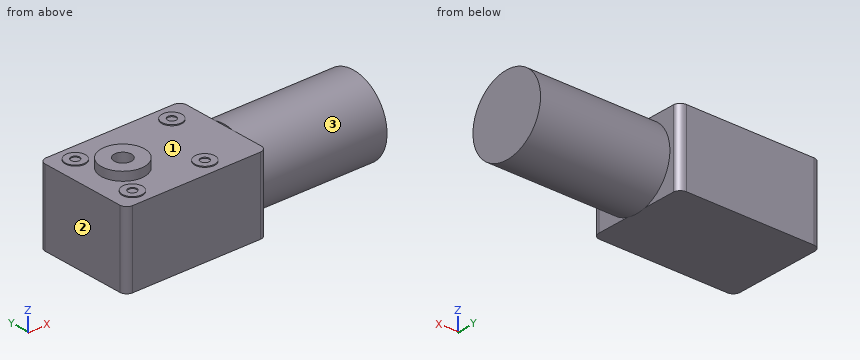
```python
from build123d import *

# Parameters (mm, degrees)
EXTRUDE_1_DEPTH     = 43.5
SKETCH_3_R          = 5.8
SKETCH_3_R_2        = 2.5
EXTRUDE_2_DEPTH     = 0.557471264
SKETCH_3_3_R        = 12.42
SKETCH_3_3_R_2      = 5
EXTRUDE_3_DEPTH     = 5
SKETCH_4_R          = 22.5
EXTRUDE_4_DEPTH     = 75
CUT_EXTRUDE_START   = -10
SKETCH_3_4_R        = 5
CUT_EXTRUDE_1_DEPTH = 10


with BuildPart() as part:
    # Sketch 2 → Extrude 1 (new body)
    with BuildSketch(Plane.XY):
        with BuildLine():
            Line((-37, 28.82), (37, 28.82))
            ThreePointArc((37, 28.82), (39.828427125, 27.648427125), (41, 24.82))
            Line((41, 24.82), (41, -24.82))
            ThreePointArc((41, -24.82), (39.828427125, -27.648427125), (37, -28.82))
            Line((37, -28.82), (-37, -28.82))
            ThreePointArc((-37, -28.82), (-39.828427125, -27.648427125), (-41, -24.82))
            Line((-41, -24.82), (-41, 24.82))
            ThreePointArc((-41, 24.82), (-39.828427125, 27.648427125), (-37, 28.82))
        make_face()
    extrude(amount=EXTRUDE_1_DEPTH)

    # Sketch 3 → Extrude 2 (add)
    # profile 1 of 4: a face of its own
    with BuildSketch(Plane.XY.offset(43.5)):
        with Locations(Location((-28.6, 19, 0), (0, 0, 180))):
            Circle(SKETCH_3_R)
        with Locations((-28.6, 19)):
            Circle(SKETCH_3_R_2, mode=Mode.SUBTRACT)
    # profile 2 of 4: a face of its own
    with BuildSketch(Plane.XY.offset(43.5)):
        with Locations(Location((-28.6, -19, 0), (0, 0, 180))):
            Circle(SKETCH_3_R)
        with Locations((-28.6, -19)):
            Circle(SKETCH_3_R_2, mode=Mode.SUBTRACT)
    # profile 3 of 4: a face of its own
    with BuildSketch(Plane.XY.offset(43.5)):
        with Locations(Location((13.4, -19, 0), (0, 0, 180))):
            Circle(SKETCH_3_R)
        with Locations((13.4, -19)):
            Circle(SKETCH_3_R_2, mode=Mode.SUBTRACT)
    # profile 4 of 4: a face of its own
    with BuildSketch(Plane.XY.offset(43.5)):
        with Locations(Location((27.4, 19, 0), (0, 0, 180))):
            Circle(SKETCH_3_R)
        with Locations((27.4, 19)):
            Circle(SKETCH_3_R_2, mode=Mode.SUBTRACT)
    extrude(amount=EXTRUDE_2_DEPTH)

    # Sketch 3_3 → Extrude 3 (add)
    with BuildSketch(Plane.XY.offset(43.5)):
        with Locations(Location((-17.6, 0, 0), (0, 0, 180))):
            Circle(SKETCH_3_3_R)
        with Locations((-17.6, 0)):
            Circle(SKETCH_3_3_R_2, mode=Mode.SUBTRACT)
    extrude(amount=EXTRUDE_3_DEPTH)

    # Sketch 4 → Extrude 4 (add)
    with BuildSketch(Plane(origin=(41, 0, 0), x_dir=(0, 0, -1), z_dir=(1, 0, 0))):
        with Locations(Location((-21.75, 0, 0), (0, 0, 194.835111582))):
            Circle(SKETCH_4_R)
    extrude(amount=EXTRUDE_4_DEPTH)

    # Sketch 3_4 → Cut-Extrude 1 (cut)
    with BuildSketch(Plane.XY.offset(43.5).offset(CUT_EXTRUDE_START)):
        with Locations((-17.6, 0)):
            Circle(SKETCH_3_4_R)
    extrude(amount=CUT_EXTRUDE_1_DEPTH, mode=Mode.SUBTRACT)


solid = part.part
```
Could you check a few things on this model? Use its own coordinates, in mm. Face numbers are marked on the shaded views. A direction names the side the tool comes from. Give positions to 0.01 mm unless a question says otherwise; leave off trailing zeros. Order: outer loops, then holes, each group sorted by start corner. A loop starts at its lowest first (then second) coordinate and runs counter-clockwise, first axis right, second up.
Q1. If I drill on line 1 along Y through (x, z) = (-28.6, 43.85); line 2 along Y through (x, z) = (-17.6, 37); line 3 along X through (y, z) = (-21, 30.5), over which ranges is the centre line in solid material (lowest first)?
Q2. I'm going to push flat-ended pins straight in: P1, Ø6, axis at x = -27, y = -19.5, coming from the +Z side; P2, Ø4, axis at x = 27.4, y = 19, coming from the -Z side; P3, Ø6, axis at x = -17.6, y = 0, coming from the +Z side. Where does each tip first touch, or does it pass through?
Q3. Suppose I cut it at C-C, the plane z = 28.5. Write out the boundary of the cut face in (x, y), and give its area (3 significant figures).
Q4. Suppose I cut it at A-A, the plane x = 27.4. Write out the boundary of the cut face in (y, z).
Q5. Suppose I cut it at D-D, the plane x = -28.6. Write out the boundary of the cut face in (y, z).
Q6. Suppose I cut it at B-B, the plane y = -19. Write out the boundary of the cut face in (x, z), and give its area (3 significant figures).
Q7. For the marked faces 1, 2 and 3, which set-ups out of +Z, -Z, +X, -X, +Y, -Y let a thin tool reach every point of the face, with its end or its side?
Solution:
1. line 1: y = -24.8 to -21.5, -16.5 to -13.2, -5.77 to 5.77, 13.2 to 16.5, 21.5 to 24.8
1. line 2: y = -28.82 to -5, 5 to 28.82
1. line 3: x = -41 to 41
2. P1: stops at z = 44.06
2. P2: stops at z = 0
2. P3: stops at z = 33.5
3. outline: (-41, -24.82) arc R4 ccw to (-37, -28.82) - (37, -28.82) arc R4 ccw to (41, -24.82) - (41, -21.46) - (116, -21.46) - (116, 21.46) - (41, 21.46) - (41, 24.82) arc R4 ccw to (37, 28.82) - (-37, 28.82) arc R4 ccw to (-41, 24.82) - close
3. area: 7,930 mm2
4. outline: (-28.82, 0) - (28.82, 0) - (28.82, 43.5) - (24.8, 43.5) - (24.8, 44.06) - (21.5, 44.06) - (21.5, 43.5) - (16.5, 43.5) - (16.5, 44.06) - (13.2, 44.06) - (13.2, 43.5) - (-28.82, 43.5) - close
5. outline: (-28.82, 0) - (28.82, 0) - (28.82, 43.5) - (24.8, 43.5) - (24.8, 44.06) - (21.5, 44.06) - (21.5, 43.5) - (16.5, 43.5) - (16.5, 44.06) - (13.2, 44.06) - (13.2, 43.5) - (5.77, 43.5) - (5.77, 48.5) - (-5.77, 48.5) - (-5.77, 43.5) - (-13.2, 43.5) - (-13.2, 44.06) - (-16.5, 44.06) - (-16.5, 43.5) - (-21.5, 43.5) - (-21.5, 44.06) - (-24.8, 44.06) - (-24.8, 43.5) - (-28.82, 43.5) - close
6. outline: (-41, 0) - (41, 0) - (41, 9.7) - (116, 9.7) - (116, 33.8) - (41, 33.8) - (41, 43.5) - (19.2, 43.5) - (19.2, 44.06) - (15.9, 44.06) - (15.9, 43.5) - (10.9, 43.5) - (10.9, 44.06) - (7.6, 44.06) - (7.6, 43.5) - (-22.8, 43.5) - (-22.8, 44.06) - (-26.1, 44.06) - (-26.1, 43.5) - (-31.1, 43.5) - (-31.1, 44.06) - (-34.4, 44.06) - (-34.4, 43.5) - (-41, 43.5) - close
6. area: 5,380 mm2
7. face 1: +Z
7. face 2: +Z, -Z, -X, +Y, -Y
7. face 3: +X
